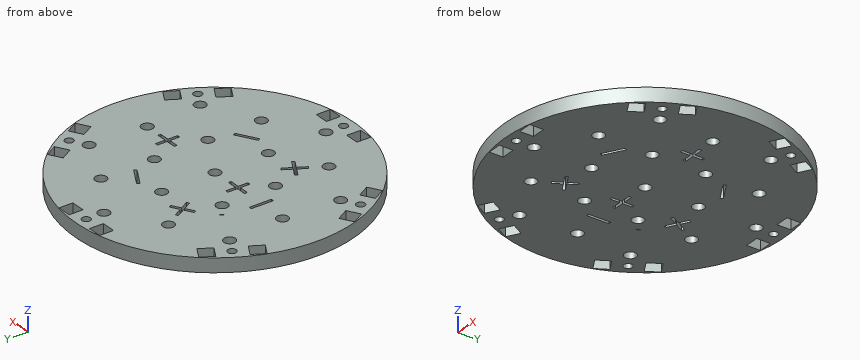
```python
from build123d import *

# Parameters (mm, degrees)
BOSS_EXTRU_1_OUTLINE_R   = 50
BOSS_EXTRU_1_OUTLINE_W   = 5
BOSS_EXTRU_1_OUTLINE_H   = 5
BOSS_EXTRU_1_OUTLINE_R_2 = 2.05
BOSS_EXTRU_1_OUTLINE_R_3 = 1.5
BOSS_EXTRU_1_DEPTH       = 5
SKETCH3_W                = 1
SKETCH3_H                = 8
CUT_EXTRUDE2_DEPTH       = 10


# Read off the part's stored shape, not the designer's step: Boss.-Extru.1
with BuildPart() as part:
    # Boss.-Extru.1 outline → Boss.-Extru.1 (new body)
    with BuildSketch(Plane.XY):
        Circle(BOSS_EXTRU_1_OUTLINE_R)
        Polygon((-37.262039705, -33.060254038), (-39.762039705, -28.730127019), (-35.431912686, -26.230127019), (-32.931912686, -30.560254038), align=None, mode=Mode.SUBTRACT)
        with Locations((-7.5, -46.3)):
            Rectangle(BOSS_EXTRU_1_OUTLINE_W, BOSS_EXTRU_1_OUTLINE_H, mode=Mode.SUBTRACT)
        with Locations((-16.666666667, -28.867513459)):
            Circle(BOSS_EXTRU_1_OUTLINE_R_2, mode=Mode.SUBTRACT)
        with Locations((-40.096976195, -23.15)):
            Circle(BOSS_EXTRU_1_OUTLINE_R_3, mode=Mode.SUBTRACT)
        Polygon((-42.931912686, -13.239745962), (-40.431912686, -17.569872981), (-44.762039705, -20.069872981), (-47.262039705, -15.739745962), align=None, mode=Mode.SUBTRACT)
        with Locations((-34.597845014, -19.975075132)):
            Circle(BOSS_EXTRU_1_OUTLINE_R_2, mode=Mode.SUBTRACT)
        with Locations((-16.671397033, -9.625235564)):
            Circle(BOSS_EXTRU_1_OUTLINE_R_2, mode=Mode.SUBTRACT)
        with Locations((0, -46.3)):
            Circle(BOSS_EXTRU_1_OUTLINE_R_3, mode=Mode.SUBTRACT)
        with Locations((7.5, -46.3)):
            Rectangle(BOSS_EXTRU_1_OUTLINE_W, BOSS_EXTRU_1_OUTLINE_H, mode=Mode.SUBTRACT)
        with Locations((0, -39.950150265)):
            Circle(BOSS_EXTRU_1_OUTLINE_R_2, mode=Mode.SUBTRACT)
        with Locations((16.666666667, -28.867513459)):
            Circle(BOSS_EXTRU_1_OUTLINE_R_2, mode=Mode.SUBTRACT)
        Polygon((32.931912686, -30.560254038), (35.431912686, -26.230127019), (39.762039705, -28.730127019), (37.262039705, -33.060254038), align=None, mode=Mode.SUBTRACT)
        with Locations((0, -19.232757636)):
            Circle(BOSS_EXTRU_1_OUTLINE_R_2, mode=Mode.SUBTRACT)
        with Locations((16.666666667, -9.622504487)):
            Circle(BOSS_EXTRU_1_OUTLINE_R_2, mode=Mode.SUBTRACT)
        with Locations((34.597845014, -19.975075132)):
            Circle(BOSS_EXTRU_1_OUTLINE_R_2, mode=Mode.SUBTRACT)
        with Locations((40.096976195, -23.15)):
            Circle(BOSS_EXTRU_1_OUTLINE_R_3, mode=Mode.SUBTRACT)
        Polygon((47.262039705, -15.739745962), (44.762039705, -20.069872981), (40.431912686, -17.569872981), (42.931912686, -13.239745962), align=None, mode=Mode.SUBTRACT)
        with Locations((-33.333333333, 0)):
            Circle(BOSS_EXTRU_1_OUTLINE_R_2, mode=Mode.SUBTRACT)
        Polygon((-47.262039705, 15.739745962), (-44.762039705, 20.069872981), (-40.431912686, 17.569872981), (-42.931912686, 13.239745962), align=None, mode=Mode.SUBTRACT)
        with Locations((-40.096976195, 23.15)):
            Circle(BOSS_EXTRU_1_OUTLINE_R_3, mode=Mode.SUBTRACT)
        with Locations((-34.597845014, 19.975075132)):
            Circle(BOSS_EXTRU_1_OUTLINE_R_2, mode=Mode.SUBTRACT)
        with Locations((-16.671397032, 9.625235564)):
            Circle(BOSS_EXTRU_1_OUTLINE_R_2, mode=Mode.SUBTRACT)
        Polygon((-32.931912686, 30.560254038), (-35.431912686, 26.230127019), (-39.762039705, 28.730127019), (-37.262039705, 33.060254038), align=None, mode=Mode.SUBTRACT)
        with Locations((-16.666666667, 28.867513459)):
            Circle(BOSS_EXTRU_1_OUTLINE_R_2, mode=Mode.SUBTRACT)
        with Locations((-7.5, 46.3)):
            Rectangle(BOSS_EXTRU_1_OUTLINE_W, BOSS_EXTRU_1_OUTLINE_H, mode=Mode.SUBTRACT)
        Circle(BOSS_EXTRU_1_OUTLINE_R_2, mode=Mode.SUBTRACT)
        with Locations((16.669571796, 9.624181764)):
            Circle(BOSS_EXTRU_1_OUTLINE_R_2, mode=Mode.SUBTRACT)
        with Locations((0, 19.165334425)):
            Circle(BOSS_EXTRU_1_OUTLINE_R_2, mode=Mode.SUBTRACT)
        with Locations((33.333333333, 0)):
            Circle(BOSS_EXTRU_1_OUTLINE_R_2, mode=Mode.SUBTRACT)
        with Locations((34.597845014, 19.975075133)):
            Circle(BOSS_EXTRU_1_OUTLINE_R_2, mode=Mode.SUBTRACT)
        Polygon((42.931912686, 13.239745962), (40.431912686, 17.569872981), (44.762039705, 20.069872981), (47.262039705, 15.739745962), align=None, mode=Mode.SUBTRACT)
        with Locations((40.096976195, 23.15)):
            Circle(BOSS_EXTRU_1_OUTLINE_R_3, mode=Mode.SUBTRACT)
        with Locations((16.666666667, 28.867513459)):
            Circle(BOSS_EXTRU_1_OUTLINE_R_2, mode=Mode.SUBTRACT)
        with Locations((0, 39.950150265)):
            Circle(BOSS_EXTRU_1_OUTLINE_R_2, mode=Mode.SUBTRACT)
        with Locations((0, 46.3)):
            Circle(BOSS_EXTRU_1_OUTLINE_R_3, mode=Mode.SUBTRACT)
        with Locations((7.5, 46.3)):
            Rectangle(BOSS_EXTRU_1_OUTLINE_W, BOSS_EXTRU_1_OUTLINE_H, mode=Mode.SUBTRACT)
        Polygon((37.262039705, 33.060254038), (39.762039705, 28.730127019), (35.431912686, 26.230127019), (32.931912686, 30.560254038), align=None, mode=Mode.SUBTRACT)
    extrude(amount=BOSS_EXTRU_1_DEPTH)

    # Sketch3 → Cut-Extrude2 (cut)
    with BuildSketch(Plane.XY.offset(5)):
        with Locations((-22.833333333, 0)):
            Rectangle(SKETCH3_W, SKETCH3_H)
        Polygon((-13.233653965, 23.921361037), (-14.099679369, 23.421361037), (-12.349679369, 20.390272124), (-15.380768282, 18.640272124), (-14.880768282, 17.77424672), (-11.849679369, 19.52424672), (-10.099679369, 16.493157806), (-9.233653965, 16.993157806), (-10.983653965, 20.02424672), (-7.952565052, 21.77424672), (-8.452565052, 22.640272124), (-11.483653965, 20.890272124), align=None)
        Polygon((15.130768282, 18.207259422), (14.630768282, 17.341234018), (7.702565052, 21.341234018), (8.202565052, 22.207259422), align=None)
        Polygon((8.202565052, -22.207259422), (7.702565052, -21.341234018), (14.630768282, -17.341234018), (15.130768282, -18.207259422), align=None)
        Polygon((27.333333333, -0.5), (27.333333333, 0.5), (23.833333333, 0.5), (23.833333333, 4), (22.833333333, 4), (22.833333333, 0.5), (19.333333333, 0.5), (19.333333333, -0.5), (22.833333333, -0.5), (22.833333333, -4), (23.833333333, -4), (23.833333333, -0.5), align=None)
        Polygon((-14.099679369, -23.421361037), (-13.233653965, -23.921361037), (-11.483653965, -20.890272124), (-8.452565052, -22.640272124), (-7.952565052, -21.77424672), (-10.983653965, -20.02424672), (-9.233653965, -16.993157806), (-10.099679369, -16.493157806), (-11.849679369, -19.52424672), (-14.880768282, -17.77424672), (-15.380768282, -18.640272124), (-12.349679369, -20.390272124), align=None)
        Polygon((-7.005935602, -0.708643072), (-7.005935602, 0.291356928), (-10.505935602, 0.291356928), (-10.505935602, 3.791356928), (-11.505935602, 3.791356928), (-11.505935602, 0.291356928), (-15.005935602, 0.291356928), (-15.005935602, -0.708643072), (-11.505935602, -0.708643072), (-11.505935602, -4.208643072), (-10.505935602, -4.208643072), (-10.505935602, -0.708643072), align=None)
        Polygon((-20.645633013, 13.413868493), (-21.300480769, 12.280855673), (-21.552183494, 12.425987884), (-20.897335737, 13.559000705), align=None)
    extrude(amount=-CUT_EXTRUDE2_DEPTH, mode=Mode.SUBTRACT)


solid = part.part
```
Geometry check sheet. Reference: the model listing, model coordinates, mm. Round coordinates to 2 decimals unless told otherwise and drop trailing zeros. Order: outer loops, then holes, each group sorted by start corner. A loop starts at its lowest first (then second) coordinate and runs counter-clockwise, first axis right, second up. Notation, with made-up numbers: (5, 3) -> (61, 3) arc R13 cw to (61, 23) -> close; hole circle Ø1 at (46.25, 12.5). An arc over 180 degrees is marked (long way). Return JSON: item names as keys, results as strings. Group by question number.
Q1. Gauge pin test, flat ends, axial feed: pin 1 (2 mm diameter, centred on y = 39.5, z = 2, fed in from -X); pin 2 (1.5 mm diameter, centred on y = -47, z = 1.5, fed in from +X); pin 3 (1.5 mm diameter, centred on y = -12.5, z = 2.5, fed in from +X). Record the tip position at first contact, or that the pin passes through.
Q2. Material ranges on probe 1 along X at (y, z) = (-14.5, 1.75); probe 2 along X at (y, z) = (-29, 4.3); probe 3 along X at (y, z) = (24, 2), recorded low to high. Write a range as from..to.
Q3. Section check A-A, the plane x = 0. Count the separate pieces of the cut face and the enclosed holes in it, plus the area to 4 significant figures.
Q4. Section check B-B, the plane y = -46.3. Record the boundary of the cut face in (x, z), plus the area to 3 significant figures.
Q5. Section check C-C, the plane x = -25.5. Record the boundary of the cut face in (y, z), plus the area to 3 significant figures.
Numbers:
{
 "1": {"pin 1": "x = -31.9", "pin 2": "x = 19", "pin 3": "x = 48.6"},
 "2": {"probe 1": "-47.85..-45.11, -42.2..42.2, 45.11..47.85", "probe 2": "-40.73..-39.61, -33.83..-18.71, -14.62..14.62, 18.71..33.83, 39.61..40.73", "probe 3": "-43.86..-41.33, -38.86..38.86, 41.33..43.86"},
 "3": {"separate pieces": "8", "enclosed holes": "0", "area": "367.5 mm^2"},
 "4": {"outline": "(-18.88, 0) -> (-10, 0) -> (-10, 5) -> (-18.88, 5) -> close; (-5, 0) -> (-1.5, 0) -> (-1.5, 5) -> (-5, 5) -> close; (1.5, 0) -> (5, 0) -> (5, 5) -> (1.5, 5) -> close; (10, 0) -> (18.88, 0) -> (18.88, 5) -> (10, 5) -> close", "area": "124 mm^2"},
 "5": {"outline": "(-43.01, 0) -> (43.01, 0) -> (43.01, 5) -> (-43.01, 5) -> close", "area": "430 mm^2"}
}
